Read the model definition and answer for the solid it produces. Units are mm, in the model's axes. Face numbers are marked on the shaded views. A direction names the side the tool comes from. Coordinates: 2 decimals unless noted, no trailing zeros. Order: outer loops, then holes, each group sorted by start corner. A loop starts at its lowest first (then second) coordinate and runs counter-clockwise, first axis right, second up. Notation, with made-up numbers: (22, -25) -> (34, -25) arc R20 ccw to (34, -17) -> close; hole circle Ø1 at (72.5, 65.5). An arc over 180 degrees is marked (long way). Use CSV: the item, a comma, the result in double quotes.
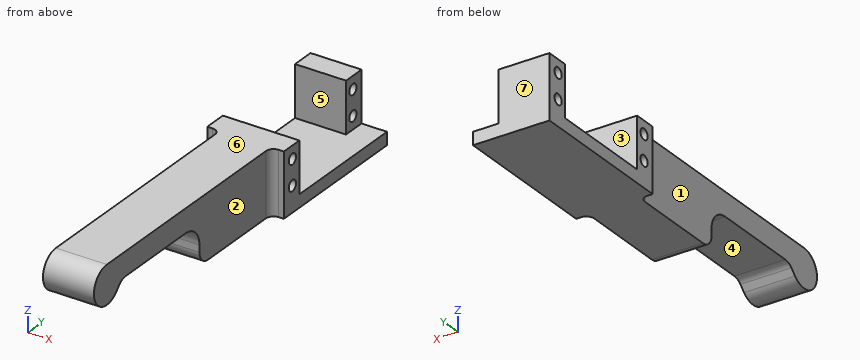
```python
from build123d import *

# Parameters (mm, degrees)
EXTRUDE_1_DEPTH     = 25
CUT_EXTRUDE_1_DEPTH = 20
SKETCH_3_R          = 2.1
CUT_EXTRUDE_2_DEPTH = 139.614573548
CUT_EXTRUDE_4_DEPTH = 138.61903938


with BuildPart() as part:
    # 草图1 → 凸台-拉伸1 (new body)
    with BuildSketch(Plane.XY):
        with BuildLine():
            Line((-15, -30), (-13, -30))
            ThreePointArc((-13, -30), (-10.878679656, -30.878679656), (-10, -33))
            Line((-10, -33), (-10, -133))
            Line((-10, -133), (0, -133))
            Line((0, -133), (10, -133))
            Line((10, -133), (10, -61))
            Line((10, -61), (10, -33))
            ThreePointArc((10, -33), (10.878679656, -30.878679656), (13, -30))
            Line((13, -30), (15, -30))
            Line((15, -30), (15, 30))
            Line((15, 30), (-15, 30))
            Line((-15, 30), (-15, -30))
        make_face()
    extrude(amount=EXTRUDE_1_DEPTH)

    # 草图2 → 切除-拉伸1 (cut)
    with BuildSketch(Plane.XY.offset(25)):
        Polygon((-15, -21), (15, -21), (15, 30), (5, 30), (5, 21), (-15, 21), align=None)
    extrude(amount=-CUT_EXTRUDE_1_DEPTH, mode=Mode.SUBTRACT)

    # 草图3 → 切除-拉伸2 (cut, through all)
    with BuildSketch(Plane.ZY.offset(15)):
        with Locations(Location((10.075, 25, 0), (0, 0, 270))):
            Circle(SKETCH_3_R)
        with Locations(Location((19.925, 25, 0), (0, 0, 270))):
            Circle(SKETCH_3_R)
        with Locations(Location((19.925, -25, 0), (0, 0, 90))):
            Circle(SKETCH_3_R)
        with Locations(Location((10.075, -25, 0), (0, 0, 90))):
            Circle(SKETCH_3_R)
    extrude(amount=-CUT_EXTRUDE_2_DEPTH, mode=Mode.SUBTRACT)

    # 草图5 → 切除-拉伸4 (cut, through all)
    with BuildSketch(Plane.ZY.offset(10)):
        with BuildLine():
            Line((12.196699141, -120.196699141), (14.267766953, -118.125631329))
            ThreePointArc((14.267766953, -118.125631329), (15.35163071, -116.503514585), (15.732233047, -114.590097423))
            Line((15.732233047, -114.590097423), (15.732233047, -79.661165235))
            ThreePointArc((15.732233047, -79.661165235), (13.389087297, -74.004310986), (7.732233047, -71.661165235))
            Line((7.732233047, -71.661165235), (5, -71.661165235))
            ThreePointArc((5, -71.661165235), (1.464466094, -70.196699141), (0, -66.661165235))
            Line((0, -66.661165235), (0, -143.423968406))
            Line((0, -143.423968406), (25, -142.592205506))
            Line((25, -142.592205506), (25, -125.5))
            ThreePointArc((25, -125.5), (14.629874257, -132.429096494), (12.196699141, -120.196699141))
        make_face()
    extrude(amount=-CUT_EXTRUDE_4_DEPTH, mode=Mode.SUBTRACT)


solid = part.part
```
Item 1: A tool of negligible diameter and unlimited length cuts with its end or side. For the marked faces 1, 2 and 3, from which of +Z, -Z, +X, -X, +Y, -Y can it reach the whole face along a straight path? Write none if from no direction.
Return value:
face 1,"+Z, -Z, -X, -Y"
face 2,"+Z, -Z, +X, -Y"
face 3,"+Z, +X, -X"
Item 2: Find section A-A, the plane y = -25. Give the vertices of the cut face in (x, z) (3 decimals), then the cut area to 3 significant figures.
Return value:
outline,"(-15, 0) -> (15, 0) -> (15, 7.975) -> (-15, 7.975) -> close; (-15, 12.175) -> (15, 12.175) -> (15, 17.825) -> (-15, 17.825) -> close; (-15, 22.025) -> (15, 22.025) -> (15, 25) -> (-15, 25) -> close"
area,"498 mm^2"
Item 3: Find section B-B, the plane x = 3.5. Give the vertices of the cut face in (y, z) (3 decimals).
Return value:
outline,"(-125.5, 25) arc R7.5 ccw (long way) to (-120.197, 12.197) -> (-118.126, 14.268) arc R5 cw to (-114.59, 15.732) -> (-79.661, 15.732) arc R8 cw to (-71.661, 7.732) -> (-71.661, 5) arc R5 ccw to (-66.661, 0) -> (30, 0) -> (30, 25) -> (21, 25) -> (21, 5) -> (-21, 5) -> (-21, 25) -> close; hole circle Ø4.2 at (-25, 10.075); hole circle Ø4.2 at (-25, 19.925); hole circle Ø4.2 at (25, 10.075); hole circle Ø4.2 at (25, 19.925)"
Item 4: The mould has two halves that part along Y. Classify the marked faces 4, 5, 6 and 7: +Y half, -Y half, draft (parallel to the pull), parting line (faces both ways), or undercut.
Return value:
face 4,"undercut"
face 5,"undercut"
face 6,"draft"
face 7,"+Y half"
Item 5: Find section D-D, the plane y = 25. Give the vertices of the cut face in (x, z) (3 decimals).
Return value:
outline,"(-15, 0) -> (15, 0) -> (15, 5) -> (5, 5) -> (5, 7.975) -> (-15, 7.975) -> close; (-15, 12.175) -> (5, 12.175) -> (5, 17.825) -> (-15, 17.825) -> close; (-15, 22.025) -> (5, 22.025) -> (5, 25) -> (-15, 25) -> close"
Item 6: Straight lines are drawn through the part: line 1 along Z through (x, y) = (-5.75, -25) (3 decimals); line 2 along Y through (x, z) = (-7.25, 11); line 3 along Y through (x, z) = (1.75, 21.75). For each, find the intervals that lie inside material, in ascending order.
Return value:
line 1,"z = 0 to 7.975, 12.175 to 17.825, 22.025 to 25"
line 2,"y = -129.24 to -121.76, -72.36 to -26.89, -23.11 to -21, 21 to 23.11, 26.89 to 30"
line 3,"y = -131.68 to -26.04, -23.96 to -21, 21 to 23.96, 26.04 to 30"
Item 7: Each of these flat-tipped pins is pushed along its axis until it touches: P1, Ø12.5, axis at y = -101.5, z = 17.5, coming from the +X side; P2, Ø1.6, axis at x = -13.5, z = 17, coming from the -Y side; P3, Ø4, axis at x = 5, y = -108, coming from the -Z side; P4, Ø3.5, axis at y = 25, z = 19.925, coming from the -X side. Where does it stop, or does it pass through?
Return value:
P1,"stops at x = 10"
P2,"stops at y = -30.02"
P3,"stops at z = 15.73"
P4,"passes through"
Item 8: Find section C-C, the plane z = 2. Give the vertices of the cut face in (x, y), then the cut area to 3 significant figures.
Return value:
outline,"(-15, -30) -> (-13, -30) arc R3 cw to (-10, -33) -> (-10, -70.66) -> (10, -70.66) -> (10, -33) arc R3 cw to (13, -30) -> (15, -30) -> (15, 30) -> (-15, 30) -> close"
area,"2,620 mm^2"
